Work out the finished part from the listing and answer in its coordinate system (mm). A direction names the side the tool comes from. Give positions to 0.01 mm unless a question says otherwise; leave off trailing zeros. Loops run counter-clockwise (first coordinate to the right, second up) from the corner with the lowest first, then second, coordinate; pieces in that order, holes last. Notation, with made-up numbers: (26.5, 47) - (57.5, 47) arc R11 ccw to (57.5, 57) - close; hole circle Ø7 at (16.25, 81). An arc over 180 degrees is marked (long way). One line per item, written item: value.
from build123d import *

# Parameters (mm, degrees)
BOSS_EXTRUDE1_DEPTH = 35
SKETCH17_W          = 133.012031184
SKETCH17_H          = 150.020262135
CUT_EXTRUDE1_DEPTH  = 100
SKETCH18_W          = 192.413181094
SKETCH18_H          = 151.943406229
CUT_EXTRUDE2_DEPTH  = 100
SKETCH19_W          = 213.02940575
SKETCH19_H          = 185.007600509
CUT_EXTRUDE3_DEPTH  = 100


with BuildPart() as part:
    # Sketch1 → Boss-Extrude1 (new body)
    with BuildSketch(Plane.XY):
        Polygon((0, 80.829037687), (-70, -40.414518843), (70, -40.414518843), align=None)
    extrude(amount=BOSS_EXTRUDE1_DEPTH)

    # Sketch17 → Cut-Extrude1 (cut)
    with BuildSketch(Plane(origin=(-14.288690166, 8.249579114, 23.333333333), x_dir=(0.8655579140838772, 0.1356024462386485, 0.4821011034429005), z_dir=(-0.5000000000000012, 0.2886751345948135, 0.8164965809277251))):
        with Locations((-15.800869145, 16.431717582)):
            Rectangle(SKETCH17_W, SKETCH17_H)
    extrude(amount=CUT_EXTRUDE1_DEPTH, mode=Mode.SUBTRACT)

    # Sketch18 → Cut-Extrude2 (cut)
    with BuildSketch(Plane(origin=(0, -16.499158228, 23.333333333), x_dir=(-0.9999855172716196, -0.004394333245699285, -0.003107262836822865), z_dir=(-3.769120432428607e-15, 0.577350269189629, -0.8164965809277238))):
        with Locations((-12.623056854, 9.892836606)):
            Rectangle(SKETCH18_W, SKETCH18_H)
    extrude(amount=-CUT_EXTRUDE2_DEPTH, mode=Mode.SUBTRACT)

    # Sketch19 → Cut-Extrude3 (cut)
    with BuildSketch(Plane(origin=(14.288690166, 8.249579114, 23.333333333), x_dir=(-0.8656985035271668, 0.1407013511718839, 0.48038446141526087), z_dir=(-0.4999999999999998, -0.288675134594816, -0.8164965809277251))):
        with Locations((-1.009116112, 24.341857859)):
            Rectangle(SKETCH19_W, SKETCH19_H)
    extrude(amount=-CUT_EXTRUDE3_DEPTH, mode=Mode.SUBTRACT)

    # Sketch2 → Cut-Revolve3 (revolve, cut)
    with BuildSketch(Plane.XY.offset(35)):
        with BuildLine():
            Line((18.146292999, 0), (-18.146292999, 0))
            ThreePointArc((-18.146292999, 0), (0, 18.146292999), (18.146292999, 0))
        make_face()
    revolve(axis=Axis((0, 0, 35), (1, 0, 0)), mode=Mode.SUBTRACT)

    # Sketch11 → Cut-Revolve7 (revolve, cut)
    with BuildSketch(Plane(origin=(-14.288690166, 8.249579114, 23.333333333), x_dir=(0.865557914083877, 0.13560244623864853, 0.48210110344290047), z_dir=(-0.5000000000000012, 0.2886751345948134, 0.816496580927725))):
        with BuildLine():
            ThreePointArc((0.3071152, -3.71281039), (6.752910141, 3.94358044), (16.277375636, 7.018177971))
            Line((16.277375636, 7.018177971), (14.668951259, 55.949737526))
            Line((14.668951259, 55.949737526), (6.673269744, 55.686912283))
            Line((6.673269744, 55.686912283), (0.3071152, -3.71281039))
        make_face()
    revolve(axis=Axis((0, 17.108489111, 28.951235667), (-2.185767015328875e-15, 0.9428090415820626, -0.33333333333333554)), mode=Mode.SUBTRACT)

    # Sketch3 → Cut-Revolve8 (revolve, cut)
    with BuildSketch(Plane(origin=(14.288690166, 8.249579114, 23.333333333), x_dir=(0.8656985035271669, -0.14070135117188398, -0.4803844614152608), z_dir=(0.4999999999999997, 0.28867513459481586, 0.8164965809277251))):
        with BuildLine():
            Line((45.996636443, -35.376806478), (48.869515746, -27.910444278))
            Line((48.869515746, -27.910444278), (-3.599712524, 1.228268839))
            ThreePointArc((-3.599712524, 1.228268839), (0.992741724, -7.712219863), (0.122393367, -17.725484464))
            Line((0.122393367, -17.725484464), (45.996636443, -35.376806478))
        make_face()
    revolve(axis=Axis((54.949625504, -31.725181077, 12.566909326), (-0.8164965809277288, 0.4714045207910254, 0.3333333333333354)), mode=Mode.SUBTRACT)

    # Sketch10 → Cut-Revolve9 (revolve, cut)
    with BuildSketch(Plane(origin=(0, -16.499158228, 23.333333333), x_dir=(0.9999855172716196, 0.004394333245699285, 0.00310726283682286), z_dir=(3.774324602856538e-15, -0.5773502691896293, 0.8164965809277237))):
        with BuildLine():
            Line((-14.763802711, 9.810092208), (-55.095676422, -18.384483489))
            Line((-55.095676422, -18.384483489), (-50.512095827, -24.941219638))
            Line((-50.512095827, -24.941219638), (3.05684637, 2.301752381))
            ThreePointArc((3.05684637, 2.301752381), (-6.936954181, 3.484349057), (-14.763802711, 9.810092208))
        make_face()
    revolve(axis=Axis((-14.81638619, -8.554244555, 28.951235667), (-0.8164965809277253, -0.471404520791033, -0.3333333333333334)), mode=Mode.SUBTRACT)

    # Sketch13 → Revolve2 (revolve)
    with BuildSketch(Plane(origin=(14.288690166, 8.249579114, 23.333333333), x_dir=(0.8656985035271668, -0.14070135117188393, -0.48038446141526087), z_dir=(0.49999999999999983, 0.2886751345948159, 0.8164965809277251))):
        with BuildLine():
            Line((9.570149417, 6.380099611), (17.89065236, 11.927101574))
            ThreePointArc((17.89065236, 11.927101574), (16.50390187, 4.993349121), (9.570149417, 6.380099611))
        make_face()
    revolve(axis=Axis((35, 20.207259422, 6.422619668), (-0.7071067811865586, -0.40824829046384215, 0.5773502691896272)))

    # Sketch14 → Cut-Revolve10 (revolve, cut)
    with BuildSketch(Plane(origin=(-14.288690166, 8.249579114, 23.333333333), x_dir=(0.865557914083877, 0.13560244623864853, 0.4821011034429005), z_dir=(-0.5000000000000013, 0.2886751345948133, 0.8164965809277251))):
        with BuildLine():
            Line((-7.635267484, 5.061697438), (-16.159640076, 10.663042982))
            ThreePointArc((-16.159640076, 10.663042982), (-14.698126552, 3.600183914), (-7.635267484, 5.061697438))
        make_face()
    revolve(axis=Axis((-35, 20.207259422, 6.422619668), (0.7077422098959172, -0.40714637457257147, 0.5773498021165807)), mode=Mode.SUBTRACT)

    # Sketch16 → Cut-Revolve11 (revolve, cut)
    with BuildSketch(Plane(origin=(0, -16.499158228, 23.333333333), x_dir=(1, 0, 0), z_dir=(3.774324602856538e-15, -0.577350269189629, 0.8164965809277237))):
        with BuildLine():
            Line((0, -21.601888146), (0, -11.401888146))
            ThreePointArc((0, -11.401888146), (5.1, -16.501888146), (0, -21.601888146))
        make_face()
    revolve(axis=Axis((0, -40.414518843, 6.422619668), (-2.2050404815138315e-15, 0.8164965809277238, 0.5773502691896291)), mode=Mode.SUBTRACT)


solid = part.part
1. For faces 5 (the flat face through (0.17, 61.78, 8.43)), 6 (the flat face through (-34.51, 21.056, 3.166)), determine the directions among +Z, -Z, +X, -X, +Y, -Y from which every point of the face is accessible in a straight line to the end or side of a thin tool.
Output:
face 5: +Z
face 6: +Z, -Z, -X, +Y
2. Flat-ended cylindrical pins translate along their axes: pin 1 Ø4 at (y, z) = (-14.5, 6) entering from -X; pin 2 Ø5 at (y, z) = (16, 6) entering from +X; pin 3 Ø3 at (x, z) = (-11, 3.5) entering from +Y. Find the tip coordinate at first contact, or state that the pin passes through.
Output:
pin 1: stops at x = -56.19
pin 2: stops at x = 38.87
pin 3: stops at y = 64.37
3. Section B-B (z = 21.5) is taken. Count the separate pieces of the cut face and the enclosed holes in it, and give its area (3 significant figures).
Output:
separate pieces: 3
enclosed holes: 0
area: 117 mm²
4. Find the intervals of material crossed by line 1 along X through (y, z) = (16, 17); line 2 along Z through (x, y) = (16.5, -24); line 3 along Y through (x, z) = (28, 13.5), in increasing order.
Output:
line 1: x = -20.03 to -8.6, 8.6 to 20.16, 22.25 to 29.67
line 2: z = 0 to 18.03
line 3: y = -30.41 to -25.88, -8.46 to 19.54
5. Section A-A (x = 61.5) is taken. Write down the section's boundary in (y, z), and give its area (3 significant figures).
Output:
outline: (-40.41, 0) - (-25.69, 0) - (-25.69, 6.42) - (-35.51, 9.89) - (-40.41, 6.42) - close
area: 120 mm²
6. The mould has two halves that part along Y. Classify faces 1 (the conical face through (26.905, -15.326, 11.077)), 2 (the flat face through (53.52, -31.16, 8.27)), 3 (the flat face through (-1, 8, 0)), 4 (the flat face through (-27.54, 17.55, 11.93)): released by +Y, released by -Y, zero draft, split by the parting line, or undercut.
Output:
face 1: undercut
face 2: undercut
face 3: zero draft
face 4: released by +Y
